Work out the finished part from the listing and answer in its coordinate system (mm). Face numbers are marked on the shaded views. A direction names the side the tool comes from. Round coordinates to 2 decimals unless told otherwise and drop trailing zeros. Order: outer loops, then holes, each group sorted by start corner. A loop starts at its lowest first (then second) coordinate and runs counter-clockwise, first axis right, second up. Notation, with made-up numbers: (-39, 79.25) - (15, 79.25) arc R26 ccw to (15, 114.25) - close; hole circle Ø3 at (1.25, 39.5). An arc over 180 degrees is marked (long way). Put each result on its own line as item: value.
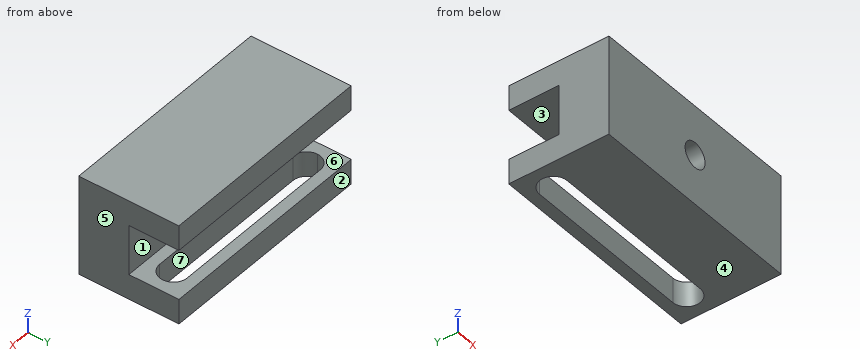
```python
from build123d import *

# Parameters (mm, degrees)
SKETCH1_W               = 44
SKETCH1_H               = 20
SKETCH1_R               = 2.55
BOSS_EXTRUDE1_DEPTH     = 7.5
SKETCH2_W               = 44
SKETCH2_H               = 20
BOSS_EXTRUDE2_DEPTH     = 2.5
SKETCH3_W               = 44
SKETCH3_H               = 5
BOSS_EXTRUDE3_DEPTH     = 10
CUT_EXTRUDE1_DEPTH      = 1
CUT_EXTRUDE1_DEPTH_BACK = 5


with BuildPart() as part:
    # Sketch1 → Boss-Extrude1 (new body)
    with BuildSketch(Plane(origin=(0, 0, 0), x_dir=(1, 0, 0), z_dir=(0, 1, 0))):
        with Locations((22, 10)):
            Rectangle(SKETCH1_W, SKETCH1_H)
        with Locations((22, 10)):
            Circle(SKETCH1_R, mode=Mode.SUBTRACT)
    extrude(amount=BOSS_EXTRUDE1_DEPTH)

    # Sketch2 → Boss-Extrude2 (add)
    with BuildSketch(Plane(origin=(0, 7.5, 0), x_dir=(1, 0, 0), z_dir=(0, 1, 0))):
        with Locations((22, 10)):
            Rectangle(SKETCH2_W, SKETCH2_H)
    extrude(amount=BOSS_EXTRUDE2_DEPTH)

    # Sketch3 → Boss-Extrude3 (add)
    with BuildSketch(Plane(origin=(0, 10, 0), x_dir=(1, 0, 0), z_dir=(0, 1, 0))):
        with Locations((22, 2.5)):
            Rectangle(SKETCH3_W, SKETCH3_H)
        with Locations((22, 17.5)):
            Rectangle(SKETCH3_W, SKETCH3_H)
    extrude(amount=BOSS_EXTRUDE3_DEPTH)

    # Sketch4 → Cut-Extrude1 (cut, two sides)
    with BuildSketch(Plane(origin=(0, 0, -20), x_dir=(-1, 0, 0), z_dir=(0, 0, -1))) as cut_extrude1_sk:
        with BuildLine():
            Line((-5, 17.75), (-39, 17.75))
            ThreePointArc((-39, 17.75), (-37.055456352, 16.944543648), (-36.25, 15))
            ThreePointArc((-36.25, 15), (-37.055456352, 13.055456352), (-39, 12.25))
            Line((-39, 12.25), (-5, 12.25))
            ThreePointArc((-5, 12.25), (-7.75, 15), (-5, 17.75))
        make_face()
        with BuildLine():
            ThreePointArc((-36.25, 15), (-37.055456352, 16.944543648), (-39, 17.75))
            Line((-39, 17.75), (-39, 12.25))
            ThreePointArc((-39, 12.25), (-37.055456352, 13.055456352), (-36.25, 15))
        make_face()
        with BuildLine():
            Line((-39, 12.25), (-39, 17.75))
            ThreePointArc((-39, 17.75), (-41.75, 15), (-39, 12.25))
        make_face()
        with BuildLine():
            ThreePointArc((-2.25, 15), (-3.055456352, 16.944543648), (-5, 17.75))
            Line((-5, 17.75), (-5, 12.25))
            ThreePointArc((-5, 12.25), (-3.055456352, 13.055456352), (-2.25, 15))
        make_face()
        with BuildLine():
            Line((-5, 12.25), (-5, 17.75))
            ThreePointArc((-5, 17.75), (-7.75, 15), (-5, 12.25))
        make_face()
    extrude(amount=CUT_EXTRUDE1_DEPTH, mode=Mode.SUBTRACT)
    extrude(cut_extrude1_sk.sketch, amount=-CUT_EXTRUDE1_DEPTH_BACK, mode=Mode.SUBTRACT)


solid = part.part
```
1) A cutting plane is placed at C-C on y = 4.5. Write down the section's boundary in (x, z).
Findings below:
outline: (0, -20) - (44, -20) - (44, 0) - (0, 0) - close; hole circle Ø5.1 at (22, -10)
2) A cutting plane is placed at D-D on y = 17. Write down the section's boundary in (x, z).
Findings below:
outline: (0, -20) - (3.11, -20) - (3.11, -15) - (0, -15) - close; (0, -5) - (44, -5) - (44, 0) - (0, 0) - close; (40.89, -20) - (44, -20) - (44, -15) - (40.89, -15) - close
3) Straight lines are drawn through the part: L1, parallel to Y at x = 9, z = -17; L2, parallel to Z at x = 22, y = 6; L3, parallel to X at y = 2.25, z = -10. For each, find the intervals that lie inside material, in ascending order. Write a range as from..to.
Findings below:
L1: y = 0..12.25, 17.75..20
L2: z = -20..-12.55, -7.45..0
L3: x = 0..19.45, 24.55..44
4) Given pin 1 Ø1.5 at (x, z) = (30.5, -5) entering from -Y; pin 2 Ø1.5 at (x, z) = (35.5, -10) entering from +Y; pin 3 Ø2.5 at (x, z) = (21, -9.5) entering from -Y, each flat-ended and moving along its own axis, determine where each tip first touches the part or whether it passes through.
Findings below:
pin 1: stops at y = 0
pin 2: stops at y = 10
pin 3: stops at y = 7.5
5) For the marked faces 5, 6 and 7, determine the directions among +Z, -Z, +X, -X, +Y, -Y from which every point of the face is accessible in a straight line to the end or side of a thin tool.
Findings below:
face 5: +Z, -Z, +X, +Y, -Y
face 6: +X, -X, +Y
face 7: -Z
6) For a pull along Z with two mould halves and no side action, classify the marked faces 1, 2, 3 and 4 as pulls with the +Z half, pulls with the -Z half, needs draft (parallel to the pull), parting line crosses it, or undercut.
Findings below:
face 1: undercut
face 2: needs draft
face 3: undercut
face 4: pulls with the -Z half
7) A cutting plane is placed at B-B on z = -15.5. Write down the section's boundary in (x, y).
Findings below:
outline: (0, 0) - (44, 0) - (44, 20) - (0, 20) - close; hole (5, 12.25) - (39, 12.25) arc R2.75 ccw to (39, 17.75) - (5, 17.75) arc R2.75 ccw to start
8) A cutting plane is placed at A-A on x = 5.5. Write down the section's boundary in (y, z).
Findings below:
outline: (0, -20) - (12.25, -20) - (12.25, -15) - (10, -15) - (10, -5) - (20, -5) - (20, 0) - (0, 0) - close; (17.75, -20) - (20, -20) - (20, -15) - (17.75, -15) - close
